Verification items for this drawing (mm, ordinates from the low corner). Give positions to 0.01 mm unless a question says otherwise; leave off trailing zeros. Order: outer loops, then holes, each group sorted by start corner. A loop starts at its lowest first (then second) coordinate and runs counter-clockwise, first axis right, second up. Notation, with made-up numbers: (27, 42.5) -> (52, 42.5) arc R22 ccw to (52, 79.5) -> close; hole circle Ø6 at (51.25, 68.5). An arc over 180 degrees is marked (long way). One line per question, with ' | ' between items.
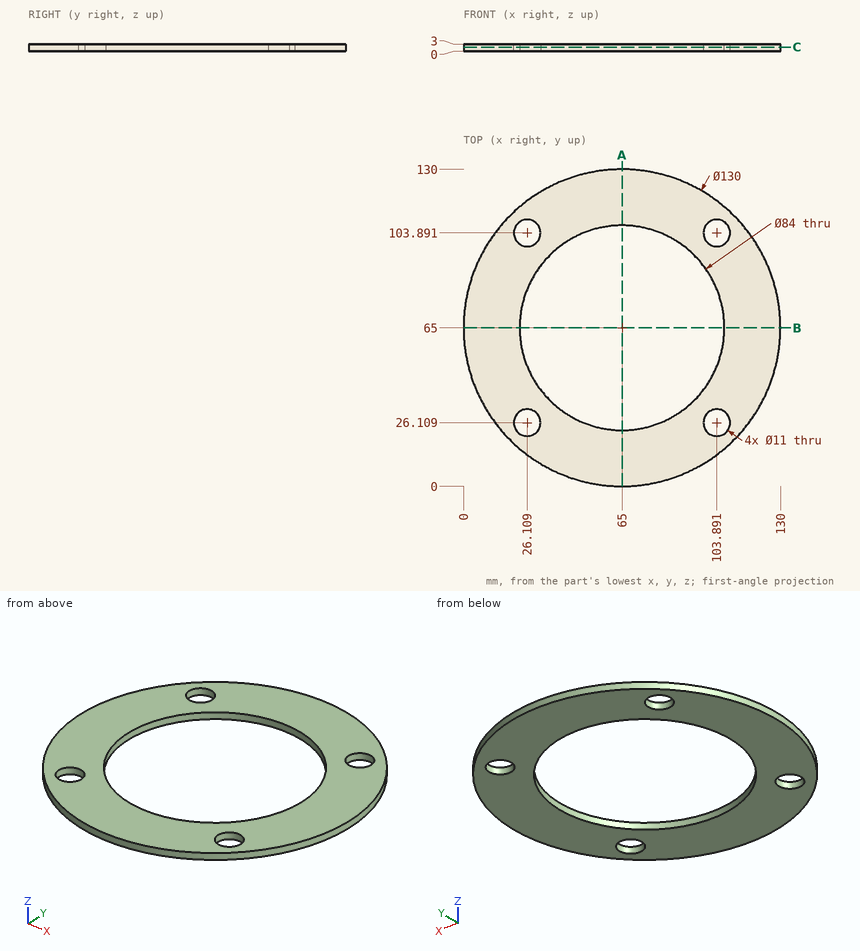
Q1. Section check A-A (x = 65). Enter the section's corners in (y, z).
Result sheet:
outline: (0, 0) -> (23, 0) -> (23, 3) -> (0, 3) -> close; (107, 0) -> (130, 0) -> (130, 3) -> (107, 3) -> close
Q2. Thickness scan on line 1 (Y direction, x = 65, z = 0.9); line 2 (X direction, y = 66, z = 1.55); line 3 (X direction, y = 99.5, z = 1.75). Record the ranges inside material, lowest first.
Result sheet:
line 1: y = 0 to 23, 107 to 130 | line 2: x = 0.01 to 23.01, 106.99 to 129.99 | line 3: x = 9.91 to 22.8, 29.42 to 41.05, 88.95 to 100.58, 107.2 to 120.09
Q3. Depth check by flat-ended pin: pin 1 Ø1.5 at (x, z) = (111.5, 2) entering from +Y. Enter the tip coordinate at first touch or a pass-through.
Result sheet:
pin 1: stops at y = 111.17
Q4. Section check C-C (z = 1.7). Enter the section's corners in (x, y), and give its area (3 significant figures).
Result sheet:
outline: circle Ø130 at (65, 65); hole circle Ø11 at (26.11, 26.11); hole circle Ø11 at (26.11, 103.89); hole circle Ø84 at (65, 65); hole circle Ø11 at (103.89, 26.11); hole circle Ø11 at (103.89, 103.89) | area: 7,350 mm2
